```python
from build123d import *

# Parameters (mm, degrees)
SKETCH1_R           = 46.395094555
BOSS_EXTRUDE1_DEPTH = 20
FILLET1_R           = 5
SKETCH2_R           = 5
CUT_EXTRUDE1_DEPTH  = 69.593072653
CUT_EXTRUDE2_DEPTH  = 69.593072653


with BuildPart() as part:
    # Sketch1 → Boss-Extrude1 (new body)
    with BuildSketch(Plane.XY):
        Circle(SKETCH1_R)
    extrude(amount=BOSS_EXTRUDE1_DEPTH)

    # Fillet1
    fillet1_edges = [part.edges().sort_by_distance(p)[0] for p in [
        (-46.395094555, 0, 0),
        (-46.395094555, 0, 20),
    ]]
    fillet(fillet1_edges, radius=FILLET1_R)

    # Sketch2 → Cut-Extrude1 (cut, through all)
    with BuildSketch(Plane.XY.offset(20)):
        Circle(SKETCH2_R)
    extrude(amount=-CUT_EXTRUDE1_DEPTH, mode=Mode.SUBTRACT)

    # Sketch3 → Cut-Extrude2 (cut, through all)
    with BuildSketch(Plane.XY.offset(20)):
        with BuildLine():
            Line((5, 10), (5, 34.891061086))
            ThreePointArc((5, 34.891061086), (13.300877708, 33.087088929), (20.104300189, 28.000604014))
            Line((20.104300189, 28.000604014), (5, 10))
        make_face()
        with BuildLine():
            Line((34.301384492, -3.410532682), (11.160254038, 0.669872981))
            Line((11.160254038, 0.669872981), (32.716545265, 13.115403524))
            ThreePointArc((32.716545265, 13.115403524), (35.304698404, 5.024646477), (34.301384492, -3.410532682))
        make_face()
        with BuildLine():
            Line((14.197084303, -31.411136696), (6.160254038, -9.330127019))
            Line((6.160254038, -9.330127019), (27.716545265, -21.775657562))
            ThreePointArc((27.716545265, -21.775657562), (22.003820696, -28.062442452), (14.197084303, -31.411136696))
        make_face()
        with BuildLine():
            Line((-20.104300189, -28.000604014), (-5, -10))
            Line((-5, -10), (-5, -34.891061086))
            ThreePointArc((-5, -34.891061086), (-13.300877708, -33.087088929), (-20.104300189, -28.000604014))
        make_face()
        with BuildLine():
            Line((-34.301384492, 3.410532682), (-11.160254038, -0.669872981))
            Line((-11.160254038, -0.669872981), (-32.716545265, -13.115403524))
            ThreePointArc((-32.716545265, -13.115403524), (-35.304698404, -5.024646477), (-34.301384492, 3.410532682))
        make_face()
        with BuildLine():
            Line((-14.197084303, 31.411136696), (-6.160254038, 9.330127019))
            Line((-6.160254038, 9.330127019), (-27.716545265, 21.775657562))
            ThreePointArc((-27.716545265, 21.775657562), (-22.003820696, 28.062442452), (-14.197084303, 31.411136696))
        make_face()
    extrude(amount=-CUT_EXTRUDE2_DEPTH, mode=Mode.SUBTRACT)


solid = part.part
```
Source: CAD feature listing. Evaluate the final solid. Frame: model axes, mm. Give positions to 0.01 mm unless a question says otherwise; leave off trailing zeros. Loops run counter-clockwise (first coordinate to the right, second up) from the corner with the lowest first, then second, coordinate; pieces in that order, holes last. Notation, with made-up numbers: M -18.5,24 L 10.5,24 A34 cw 10.5,61 Z; hole C 34.25,38.5 d8. An arc over 180 degrees is marked long. Put each result on its own line as item: value.
Q1. Section B-B (x = 0). Return the cut outline in (y, z), and give its area (3 significant figures).
Response values:
outline: M -46.4,5 A5 ccw -41.4,0 L -5,0 L -5,20 L -41.4,20 A5 ccw -46.4,15 Z; M 5,0 L 41.4,0 A5 ccw 46.4,5 L 46.4,15 A5 ccw 41.4,20 L 5,20 Z
area: 1,630 mm²
Q2. Mould query, pull axis X, two halves, no side actions, for faces 1 (the cylindrical face through (-6.04, 46, 9.93)), 2 (the flat face through (-1, -9, 0)), 3 (the cylindrical face through (-13.192, -33.136, 10.14)). Classes: released by +X, released by -X, zero draft, split by the parting line, or undercut.
Response values:
face 1: split by the parting line
face 2: zero draft
face 3: undercut
Q3. Line query: probe 1 along Y at (x, z) = (17, 3.25); probe 2 along Y at (x, z) = (-17, 8); probe 3 along X at (y, z) = (-4, 5). Output: solid intervals per line, ascending. Write a range as [from, to].
Response values:
probe 1: y = [-42.83, -30.65], [-15.59, -0.36], [4.04, 24.3], [30.89, 42.83]
probe 2: y = [-43.17, -30.89], [-24.3, -4.04], [0.36, 15.59], [30.65, 43.17]
probe 3: x = [-46.22, -35.38], [-16.93, -3], [3, 46.22]
Q4. Section A-A (z = 6.75). Return the cut outline in (x, y), and give its area (3 significant figures).
Response values:
outline: C 0,0 d92.79; hole M -34.3,3.41 A20 ccw -32.72,-13.12 L -11.16,-0.67 Z; hole M -27.72,21.78 L -6.16,9.33 L -14.2,31.41 A20 ccw Z; hole M -20.1,-28 A20 ccw -5,-34.89 L -5,-10 Z; hole C 0,0 d10; hole M 5,10 L 20.1,28 A20 ccw 5,34.89 Z; hole M 6.16,-9.33 L 14.2,-31.41 A20 ccw 27.72,-21.78 Z; hole M 11.16,0.67 L 34.3,-3.41 A20 ccw 32.72,13.12 Z
area: 5,430 mm²
Q5. Pin query (flat end, axial travel): P1, Ø4, axis at y = -23.5, z = 14.5, coming from the +X side; P2, Ø4, axis at x = -28.5, z = 11.5, coming from the -Y side; P3, Ø5, axis at y = -29, z = 2, coming from the +X side; P4, Ø3, axis at x = -21.5, y = -3, coming from the +Z side. Return the tip coordinate at first contact, or that it passes through.
Response values:
P1: stops at x = 41.11
P2: stops at y = -38.08
P3: stops at x = 37.46
P4: passes through
Q6. Section C-C (x = 24.5). Count the separate pieces of the cut face and the enclosed holes in it, and give its area (3 significant figures).
Response values:
separate pieces: 3
enclosed holes: 0
area: 1,230 mm²
